from build123d import *

# Parameters (mm, degrees)
F1_DEPTH = 1.5


with BuildPart() as f1:
    # F0 (on Top) → F1 (new body)
    with BuildSketch(Plane.XY):
        Polygon((35, 50), (0, 0), (40, 0), (40, 50), align=None)
        Polygon((9.603278, 5), (35, 41.281032), (35, 5), align=None, mode=Mode.SUBTRACT)
        Polygon((40, 0), (0, 0), (0, -40), align=None)
        Polygon((5, -27.928932), (5, -5), (27.928932, -5), align=None, mode=Mode.SUBTRACT)
    extrude(amount=F1_DEPTH)


solid = f1.part
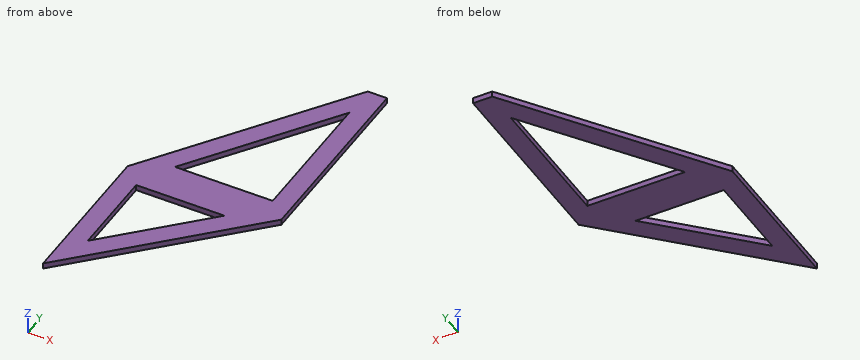
Build history of the part. All positions in model axes, mm. Coordinates: 2 decimals unless noted, no trailing zeros. Write each loop counter-clockwise with the first axis right and the second up, starting at its lowest first coordinate (ties: lowest second). Pieces come first, ordered by that corner, then holes.
(1) Cut at A-A on z = 0.8. List the corners of the cut face in (x, y), and give its area (3 significant figures).
(2) Cut at C-C on x = 8. List the corners of the cut face in (y, z).
(3) Cut at B-B on y = -8. List the corners of the cut face in (x, z), and give its area (3 significant figures).
(4) Pin check, flat tips, straight feed: pin 1 Ø0.8 at (x, z) = (20.5, 1) entering from +Y; pin 2 Ø0.8 at (x, z) = (19.5, 1) entering from -Y; pin 3 Ø0.8 at (y, z) = (-11, 1) entering from +X. Stop position of each tip, or through.
(5) Cut at D-D on x = 22.5. List the corners of the cut face in (y, z).
(6) Drill centre lines: line 1 (Y direction, x = 26.5, z = 0.75); line 2 (Y direction, x = 22, z = 0.1); line 3 (X direction, y = -25.5, z = 0.2). Where is each one in solid material? Low to high.
Working result:
1. outline: (0, -40) - (40, 0) - (40, 50) - (35, 50) - (0, 0) - close; hole (5, -27.93) - (27.93, -5) - (5, -5) - close; hole (9.6, 5) - (35, 5) - (35, 41.28) - close
1. area: 1,200 mm2
2. outline: (-32, 0) - (-24.93, 0) - (-24.93, 1.5) - (-32, 1.5) - close; (-5, 0) - (11.43, 0) - (11.43, 1.5) - (-5, 1.5) - close
3. outline: (0, 0) - (5, 0) - (5, 1.5) - (0, 1.5) - close; (24.93, 0) - (32, 0) - (32, 1.5) - (24.93, 1.5) - close
3. area: 18.1 mm2
4. pin 1: stops at y = 29.86
4. pin 2: stops at y = -20.9
4. pin 3: stops at x = 29.4
5. outline: (-17.5, 0) - (-10.43, 0) - (-10.43, 1.5) - (-17.5, 1.5) - close; (-5, 0) - (5, 0) - (5, 1.5) - (-5, 1.5) - close; (23.42, 0) - (32.14, 0) - (32.14, 1.5) - (23.42, 1.5) - close
6. line 1: y = -13.5 to -6.43, -5 to 5, 29.14 to 37.86
6. line 2: y = -18 to -10.93, -5 to 5, 22.71 to 31.43
6. line 3: x = 0 to 5, 7.43 to 14.5
